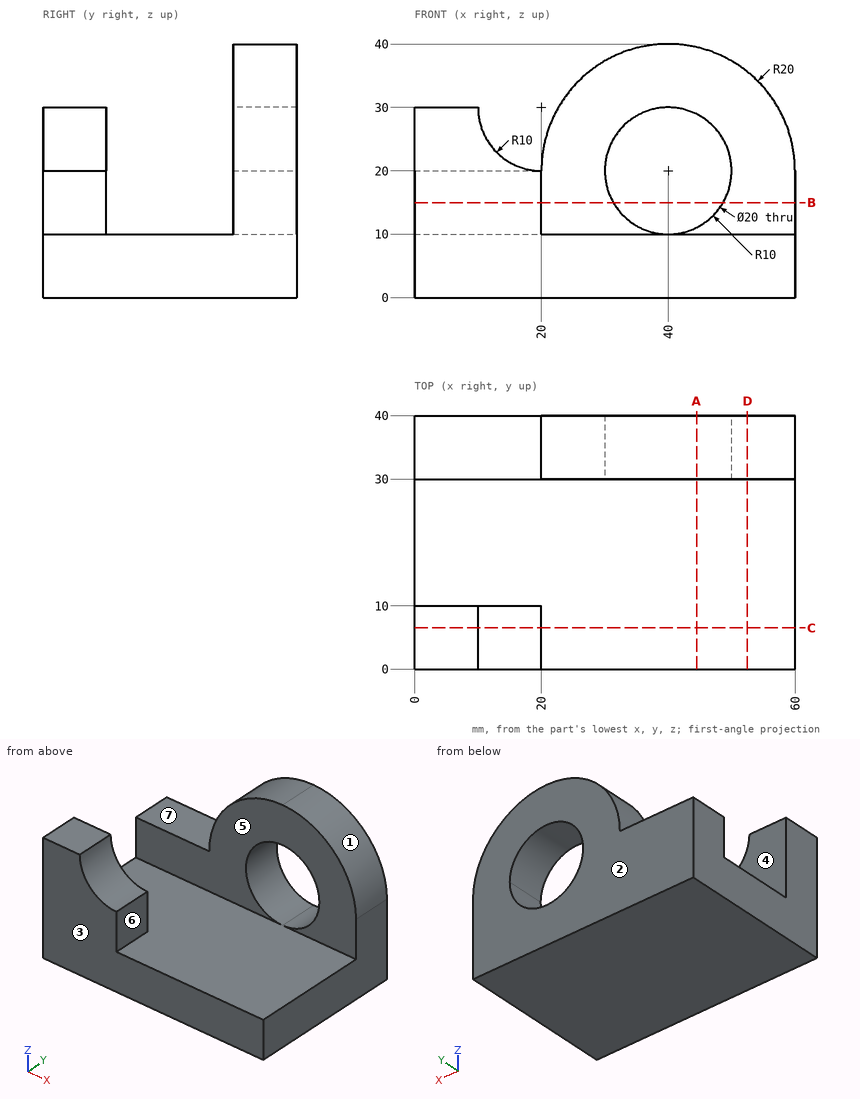
Geometry check sheet. Reference: drawing and pictorial views, mm from the part's lowest x, y, z. A direction names the side the tool comes from. Round coordinates to 2 decimals unless told otherwise and drop trailing zeros. Loops run counter-clockwise (first coordinate to the right, second up) from the corner with the lowest first, then second, coordinate; pieces in that order, holes last. Notation, with made-up numbers: (-25, 26.5) -> (11, 26.5) arc R13 cw to (11, 37.5) -> close; hole circle Ø8 at (-8, -20.75). An arc over 180 degrees is marked (long way). Answer as a JSON object with one key per item and string values.
Q1. Section check D-D (x = 52.5). Record the boundary of the cut face in (y, z), then the cut area to 3 significant figures.
Data:
{"outline": "(0, 0) -> (40, 0) -> (40, 35.61) -> (30, 35.61) -> (30, 10) -> (0, 10) -> close", "area": "656 mm2"}
Q2. Section check B-B (z = 15). Record the boundary of the cut face in (x, y).
Data:
{"outline": "(0, 0) -> (20, 0) -> (20, 10) -> (0, 10) -> close; (0, 30) -> (31.34, 30) -> (31.34, 40) -> (0, 40) -> close; (48.66, 30) -> (60, 30) -> (60, 40) -> (48.66, 40) -> close"}
Q3. Draft check along Y on the marked faces 1, 2, 3 and 4. Enter one of: pulls with the +Y half, pulls with the -Y half, needs draft (parallel to the pull), parting line crosses it, or undercut.
Data:
{"face 1": "needs draft", "face 2": "pulls with the +Y half", "face 3": "pulls with the -Y half", "face 4": "undercut"}
Q4. Section check C-C (y = 6.5). Record the boundary of the cut face in (x, z), then the cut area to 3 significant figures.
Data:
{"outline": "(0, 0) -> (60, 0) -> (60, 10) -> (20, 10) -> (20, 20) arc R10 cw to (10, 30) -> (0, 30) -> close", "area": "921 mm2"}
Q5. Access from +Z, -Z, +X, -X, +Y, -Y to the whole of each face (thin tool, end or side, straight path). Record for the marked faces 5, 6 and 7.
Data:
{"face 5": "+Z, +X, -X, -Y", "face 6": "+Z, +X, -Y", "face 7": "+Z, -X, +Y"}
Q6. Scan lines: line 1 (Z direction, x = 40, y = 35); line 2 (Y direction, x = 51, z = 22); line 3 (Z direction, x = 50, y = 25). Record each from-to range of solid material in increasing order. Write a range as from..to.
Data:
{"line 1": "z = 0..10, 30..40", "line 2": "y = 30..40", "line 3": "z = 0..10"}
Q7. Section check A-A (x = 44.5). Record the boundary of the cut face in (y, z).
Data:
{"outline": "(0, 0) -> (40, 0) -> (40, 11.07) -> (30, 11.07) -> (30, 10) -> (0, 10) -> close; (30, 28.93) -> (40, 28.93) -> (40, 39.49) -> (30, 39.49) -> close"}
Q8. Go/stop test with flat-tipped pins: P1, Ø11, axis at x = 7.5, y = 3, coming from the +Z side; P2, Ø9, axis at x = 23.5, z = 27, coming from the -Y side; P3, Ø11, axis at x = 11.5, y = 37, coming from the +Z side; P4, Ø16, axis at x = 40, z = 20, coming from the +Y side. Record where each tip stops, or that it passes through.
Data:
{"P1": "stops at z = 30", "P2": "stops at y = 30", "P3": "stops at z = 20", "P4": "passes through"}
